```python
from build123d import *

# Parameters (mm, degrees)
SKETCH069_W             = 50
SKETCH069_H             = 70
SKETCH069_R             = 6
PAD033_DEPTH            = 3
SKETCH068_W             = 20
SKETCH068_H             = 25
PAD034_DEPTH            = 12.5
SKETCH067_W             = 40
SKETCH067_H             = 33
POCKET027_DEPTH         = 5.5
FILLET_R                = 8
CHAMFER001_SIZE         = 1
BODY014_PLACEMENT_ANGLE = 210


with BuildPart() as part:
    # Sketch069 → Pad033 (new body)
    with BuildSketch(Plane.XY):
        with Locations((0, 5)):
            Rectangle(SKETCH069_W, SKETCH069_H)
        with Locations((-12.5, 27.5)):
            Circle(SKETCH069_R, mode=Mode.SUBTRACT)
        with Locations((12.5, 27.5)):
            Circle(SKETCH069_R, mode=Mode.SUBTRACT)
        with Locations((-12.5, -17.5)):
            Circle(SKETCH069_R, mode=Mode.SUBTRACT)
        with Locations((12.5, -17.5)):
            Circle(SKETCH069_R, mode=Mode.SUBTRACT)
    extrude(amount=-PAD033_DEPTH)

    # Sketch068 → Pad034 (join, symmetric)
    with BuildSketch(Plane.YZ):
        with Locations((0, 12.5)):
            Rectangle(SKETCH068_W, SKETCH068_H)
        Polygon((2.6, 10.496668), (5.2, 15), (2.6, 19.503332), (-2.6, 19.503332), (-5.2, 15), (-2.6, 10.496668), align=None, mode=Mode.SUBTRACT)
    extrude(amount=PAD034_DEPTH, both=True)

    # Sketch067 → Pocket027 (cut, symmetric)
    with BuildSketch(Plane.YZ):
        with Locations((0, 18.5)):
            Rectangle(SKETCH067_W, SKETCH067_H)
    extrude(amount=POCKET027_DEPTH, both=True, mode=Mode.SUBTRACT)

    # Fillet
    fillet_edges = [part.edges().sort_by_distance(p)[0] for p in [
        (-25, -30, -1.5),
        (-25, 40, -1.5),
        (25, 40, -1.5),
        (25, -30, -1.5),
        (-9, 10, 25),
        (9, 10, 25),
        (-9, -10, 25),
        (9, -10, 25),
    ]]
    fillet(fillet_edges, radius=FILLET_R)

    # Chamfer001
    chamfer001_edges = [part.edges().sort_by_distance(p)[0] for p in [
        (12.5, 0, 0),
        (-12.5, 0, 0),
    ]]
    chamfer(chamfer001_edges, length=CHAMFER001_SIZE)


with BuildPart() as part_1:
    # Body014 placement: moved
    add(part.part.moved(Location((-66, 77.285671, 90.10746))).rotate(Axis((-66, 77.285671, 90.10746), (1, 0, 0)), BODY014_PLACEMENT_ANGLE))


solid = part_1.part
```
Check sheet for the modelled part. Datum: model origin and axes. Units: mm. A direction names the side the tool comes from. Coordinates: 2 decimals unless noted, no trailing zeros. Loops run counter-clockwise (first coordinate to the right, second up) from the corner with the lowest first, then second, coordinate; pieces in that order, holes last.
1) Gauge pin test, flat ends, axial feed: pin 1 (5.5 mm diameter, centred on x = -74, z = 77, fed in from +Y); pin 2 (2.5 mm diameter, centred on x = -76, z = 77, fed in from -Y); pin 3 (4 mm diameter, centred on x = -75, z = 89.5, fed in from +Y); pin 4 (1 mm diameter, centred on y = 60, z = 77.5, fed in from +X). Record the tip position at first contact, or that the pin passes through.
2) Sectioned sample at B-B (z = 88). Record the boundary of the cut face in (x, y).
3) Sectioned sample at A-A (x = -58). Record the boundary of the cut face in (y, z).
4) Access from +Z, -Z, +X, -X, +Y, -Y to the whole of each face (thin tool, end or side, straight path). Record for faces 5 (the face through (-56.95, 82.57, 81.04)), 6 (the face through (-78.5, 81, 83)), 7 (the face through (-53.5, 81, 83)), 8 (the face through (-57.049, 95.267, 74.4)).
5) Sectioned sample at C-C (y = 61). Record the boundary of the cut face in (x, z).
6) Material ranges on probe 1 along Y at (x, z) = (-74.5, 80); probe 2 along X at (y, z) = (79, 69); probe 3 along Z at (x, y) = (-56.5, 89), recorded low to high.
7) Release check for a two-part mould opening along Z. For faces 1 (the face through (-71.811, 72.816, 77.849)), 2 (the face through (-56.951, 82.502, 73.235)), 3 (the face through (-84.494, 91.473, 100.006)), 4 (the face through (-88.72, 100.42, 105.22)) record: released by +Z, released by -Z, zero draft, split by the parting line, or undercut.
Check sheet entries:
1. pin 1: stops at y = 95.52
1. pin 2: stops at y = 46.42
1. pin 3: stops at y = 90.34
1. pin 4: passes through
2. outline: (-91, 67.64) - (-41, 67.64) - (-41, 73.64) - (-52.5, 73.64) - (-53.5, 75.64) - (-53.5, 90.05) - (-60.5, 90.05) - (-60.5, 77.64) - (-71.5, 77.64) - (-71.5, 90.05) - (-78.5, 90.05) - (-78.5, 75.64) - (-79.5, 73.64) - (-91, 73.64) - close
3. outline: (41.14, 72.71) - (42.64, 70.11) - (50.03, 74.37) - (48.53, 76.97) - close; (55.41, 80.94) - (56.91, 78.34) - (68.63, 85.11) - (77.13, 70.39) arc R8 ccw to (88.05, 67.46) - (91.52, 69.46) arc R8 ccw to (94.45, 80.39) - (85.95, 95.11) - (89, 96.87) - (87.5, 99.47) - close; (94.38, 103.44) - (95.88, 100.84) - (103.27, 105.11) - (101.77, 107.71) - close; hole (80.28, 74.52) - (84.79, 71.92) - (89.29, 74.52) - (89.29, 79.72) - (84.79, 82.32) - (80.28, 79.72) - close
4. face 5: +X, -X
4. face 6: -Z, -X, +Y
4. face 7: -Z, +X, +Y
4. face 8: +X, -X, +Y
5. outline: (-91, 80.7) - (-41, 80.7) - (-41, 84.17) - (-91, 84.17) - close
6. probe 1: y = 56.53 to 59.78, 71.57 to 80.77, 88.8 to 94.65
6. probe 2: x = -78.5 to -71.5, -60.5 to -53.5
6. probe 3: z = 68 to 74.35, 79.88 to 89.82
7. face 1: released by -Z
7. face 2: undercut
7. face 3: undercut
7. face 4: released by +Z
